Work out the finished part from the listing and answer in its coordinate system (mm). A direction names the side the tool comes from. Coordinates: 2 decimals unless noted, no trailing zeros. Order: outer loops, then holes, each group sorted by start corner. A loop starts at its lowest first (then second) coordinate and runs counter-clockwise, first axis right, second up. Notation, with made-up numbers: (36, 12.25) - (85, 12.25) arc R11 ccw to (85, 18.25) - close; hole circle Ø9 at (-39, 62.5). An arc over 180 degrees is marked (long way). Use CSV: the item, a comma, the result in double quotes. Start each with the question number.
from build123d import *

# Parameters (mm, degrees)
F1_DEPTH = 76.2
F3_DEPTH = 62.23


with BuildPart() as f1:
    # F0 (on Top) → F1 (new body)
    with BuildSketch(Plane.XY):
        Polygon((94.227217, 44.845942), (-35.218999, 53.311478), (-95.495798, 145.953357), (-71.593605, 44.845942), (-152.917683, 76.2394), (-80.585986, -14.665665), (-102.024987, -76.140255), (0, -83.673872), (71.544036, -172.317266), (18.6927, -21.068443), align=None)
    extrude(amount=F1_DEPTH)

    # F2 (on face) → F3 (cut)
    with BuildSketch(Plane.XY.offset(76.2)):
        Polygon((5.911248, -72.394553), (38.253499, -112.466753), (5.055551, -17.461575), (65.213298, 35.034437), (-41.821007, 42.034277), (-68.682796, 83.319259), (-55.123725, 25.963743), (-116.983429, 49.843387), (-67.43257, -12.431166), (-85.978236, -65.60935), align=None)
    extrude(amount=-F3_DEPTH, mode=Mode.SUBTRACT)


solid = f1.part
1) For faces 1 (the face through (-91.155, -44.973, 37.567)), 2 (the face through (-92.555, 19.142, 45.521)), 3 (the face through (-51.727, -79.854, 37.567)), 4 (the face through (55.9, 11.4, 37.6)), 5 (the face through (16, -12, 76.2)), determine the directions among +Z, -Z, +X, -X, +Y, -Y from which every point of the face is accessible in a straight line to the end or side of a thin tool.
2) Straight lines are drawn through the part: line 1 (Y direction, x = -4, z = 21); line 2 (Y direction, x = -42.5, z = 25.5); line 3 (X direction, y = -73.5, z = 38). For each, find the intervals that lie inside material, in ascending order. Write a range as [from, to].
3) The part is cut by section D-D on y = -5. Determine the outline of the cut face in (x, z), plus the area to 3 significant figures.
4) Flat-ended cylindrical pins translate along their axes: P1, Ø3, axis at x = -77.5, z = 50, coming from the +Y side; P2, Ø8, axis at y = -108.5, z = 62, coming from the -X side; P3, Ø10, axis at x = -49, y = -52, coming from the +Z side. Find the tip coordinate at first contact, or state that the pin passes through.
5) For a pull along X with two mould halves and no side action, classify faces 6 (the face through (34.713, 8.419, 45.521)), 7 (the face through (-76.576, -38.648, 45.521)), 8 (the face through (30.41, 49.02, 37.57)), 9 (the face through (-30, -1, 0)) as +X half, -X half, draft (parallel to the pull), parting line (faces both ways), or undercut.
6) The part is cut by section C-C on x = -23.5. Determine the outline of the cut face in (y, z).
7) The part is cut by section B-B on z = 6.5. Determine the outline of the cut face in (x, y).
8) The part is cut by section A-A on z = 66. Determine the outline of the cut face in (x, y), plus the area to 3 significant figures.
Answer key:
1,face 1,"+Z, -Z, -X"
1,face 2,"+Z"
1,face 3,"+Z, -Z, -X, -Y"
1,face 4,"+Z, -Z, +X"
1,face 5,"+Z, +X, -X, +Y, -Y"
2,line 1,"[-83.38, -71.66], [39.56, 51.27]"
2,line 2,"[-80.54, -68.82], [43.08, 64.5]"
2,line 3,"[-101.1, 6.8], [24.64, 37.01]"
3,outline,"(-88.28, 0) - (37.11, 0) - (37.11, 76.2) - (19.34, 76.2) - (19.34, 13.97) - (-73.35, 13.97) - (-73.35, 76.2) - (-88.28, 76.2) - close"
3,area,"3,790 mm^2"
4,P1,"y = 120.6"
4,P2,"x = 16.81"
4,P3,"z = 13.97"
5,face 6,"undercut"
5,face 7,"undercut"
5,face 8,"+X half"
5,face 9,"draft"
6,outline,"(-81.94, 0) - (52.55, 0) - (52.55, 76.2) - (40.84, 76.2) - (40.84, 13.97) - (-70.22, 13.97) - (-70.22, 76.2) - (-81.94, 76.2) - close"
7,outline,"(-152.92, 76.24) - (-80.59, -14.67) - (-102.02, -76.14) - (0, -83.67) - (71.54, -172.32) - (18.69, -21.07) - (94.23, 44.85) - (-35.22, 53.31) - (-95.5, 145.95) - (-71.59, 44.85) - close"
8,outline,"(-152.92, 76.24) - (-80.59, -14.67) - (-102.02, -76.14) - (0, -83.67) - (71.54, -172.32) - (18.69, -21.07) - (94.23, 44.85) - (-35.22, 53.31) - (-95.5, 145.95) - (-71.59, 44.85) - close; hole (-116.98, 49.84) - (-67.43, -12.43) - (-85.98, -65.61) - (5.91, -72.39) - (38.25, -112.47) - (5.06, -17.46) - (65.21, 35.03) - (-41.82, 42.03) - (-68.68, 83.32) - (-55.12, 25.96) - close"
8,area,"10,700 mm^2"
